Can you work these out from the model? Positions are in its coordinate system, mm. A direction names the side the tool comes from. Round coordinates to 2 decimals unless told otherwise and drop trailing zeros. Loops run counter-clockwise (first coordinate to the right, second up) from the corner with the lowest first, then second, coordinate; pieces in that order, holes last. Notation, with made-up numbers: (30.5, 20.25) -> (89.5, 20.25) arc R28 ccw to (89.5, 47.25) -> close; hole circle Ø6 at (-12.75, 51.25). An arc over 180 degrees is marked (long way). Use a Markdown table: item, result.
from build123d import *

# Parameters (mm, degrees)
PAD_DEPTH       = 86
SKETCH001_W     = 59.039818
SKETCH001_H     = 57
POCKET_DEPTH    = 56.001
SKETCH002_W     = 74.051056
SKETCH002_H     = 10
SKETCH002_W_2   = 70.317291
POCKET001_DEPTH = 51
SKETCH003_R     = 1.5
POCKET002_DEPTH = 5.001
SKETCH005_R     = 20
POCKET003_DEPTH = 30.001
SKETCH006_R     = 2.5
POCKET004_DEPTH = 30.001


with BuildPart() as part:
    # Sketch → Pad (new body)
    with BuildSketch(Plane.XZ):
        Polygon((0, 0), (30, 0), (30, 5), (5, 56), (0, 56), align=None)
    extrude(amount=PAD_DEPTH)

    # Sketch001 (on Face4 of Pad) → Pocket (cut, through all)
    with BuildSketch(Plane(origin=(0, 0, 56), x_dir=(-1, 0, 0), z_dir=(0, 0, 1))):
        with Locations((-34.519909, 43)):
            Rectangle(SKETCH001_W, SKETCH001_H)
    extrude(amount=-POCKET_DEPTH, mode=Mode.SUBTRACT)

    # Sketch002 (on Face11 of Pocket) → Pocket001 (cut)
    with BuildSketch(Plane(origin=(0, 0, 56), x_dir=(-1, 0, 0), z_dir=(0, 0, 1))):
        with Locations((-37.025528, 81)):
            Rectangle(SKETCH002_W, SKETCH002_H)
        with Locations((-35.158645, 5)):
            Rectangle(SKETCH002_W_2, SKETCH002_H)
    extrude(amount=-POCKET001_DEPTH, mode=Mode.SUBTRACT)

    # Sketch003 (on Face14 of Pocket001) → Pocket002 (cut, through all)
    with BuildSketch(Plane(origin=(0, 0, 5), x_dir=(-1, 0, 0), z_dir=(0, 0, 1))):
        with Locations((-20, 81)):
            Circle(SKETCH003_R)
        with Locations((-7.5, 81)):
            Circle(SKETCH003_R)
        with Locations((-20, 5)):
            Circle(SKETCH003_R)
        with Locations((-7.5, 5)):
            Circle(SKETCH003_R)
    extrude(amount=-POCKET002_DEPTH, mode=Mode.SUBTRACT)

    # Sketch005 (on Face3 of Pocket002) → Pocket003 (cut, through all)
    with BuildSketch(Plane(origin=(0, 0, 0), x_dir=(0, 0, -1), z_dir=(-1, 0, 0))):
        with Locations((-28, 43)):
            Circle(SKETCH005_R)
    extrude(amount=-POCKET003_DEPTH, mode=Mode.SUBTRACT)

    # Sketch006 (on Face3 of Pocket003) → Pocket004 (cut, through all)
    with BuildSketch(Plane(origin=(0, 0, 0), x_dir=(0, 0, -1), z_dir=(-1, 0, 0))):
        with Locations((-51.5, 66.5)):
            Circle(SKETCH006_R)
        with Locations((-4.5, 66.5)):
            Circle(SKETCH006_R)
        with Locations((-51.5, 19.5)):
            Circle(SKETCH006_R)
        with Locations((-4.5, 19.5)):
            Circle(SKETCH006_R)
    extrude(amount=-POCKET004_DEPTH, mode=Mode.SUBTRACT)


solid = part.part
1. Which directions (+Z, -Z, +X, -X, +Y, -Y) give clear straight access to the entire face, cutting with the end or side of a thin tool? Please do faces 5 (the flat face through (15, -14.5, 22)), 6 (the cylindrical face through (20.195, -82.487, 2.535)), 7 (the flat face through (9, -10, 25)).
Answer sheet:
| item | result |
|---|---|
| face 5 | +Z, -Z, +X |
| face 6 | +Z, -Z |
| face 7 | +Z, +X, -X, +Y |
2. I want a section at B-B (y = -43). Please give me the cut outline in (x, z), plus the area to 3 significant figures.
Answer sheet:
| item | result |
|---|---|
| outline | (0, 0) -> (5, 0) -> (5, 8) -> (0, 8) -> close; (0, 48) -> (5, 48) -> (5, 56) -> (0, 56) -> close |
| area | 80.0 mm² |
3. If we mould it in two halves opening along Z, with no side actions, what happens to faces 1 (the cylindrical face through (2.465, -49.007, 8.924)), 2 (the flat face through (17.675, -12.218, 30.143)), 3 (the flat face through (15, -71.5, 22)), 4 (the cylindrical face through (2.46, -65.54, 49.19))? For each: +Z half, -Z half, draft (parallel to the pull), parting line (faces both ways), or undercut.
Answer sheet:
| item | result |
|---|---|
| face 1 | undercut |
| face 2 | +Z half |
| face 3 | draft |
| face 4 | undercut |
4. I need wall thicknesses on line 1 (Y direction, x = 20, z = 2); line 2 (Y direction, x = 1.75, z = 51.5); line 3 (Y direction, x = 2.2, z = 4.5). Which ranges of each line are inside material? Lowest first, please.
Answer sheet:
| item | result |
|---|---|
| line 1 | y = -86 to -82.5, -79.5 to -71.5, -14.5 to -6.5, -3.5 to 0 |
| line 2 | y = -76 to -69, -64 to -22, -17 to -10 |
| line 3 | y = -86 to -69, -64 to -22, -17 to 0 |
5. I want a section at A-A (x = 15.5). Please give me the cut outline in (y, z).
Answer sheet:
| item | result |
|---|---|
| outline | (-86, 0) -> (-71.5, 0) -> (-71.5, 34.58) -> (-76, 34.58) -> (-76, 5) -> (-86, 5) -> close; (-14.5, 0) -> (0, 0) -> (0, 5) -> (-10, 5) -> (-10, 34.58) -> (-14.5, 34.58) -> close |
6. I want a section at C-C (y = -5). Please give me the cut outline in (x, z), plus the area to 3 significant figures.
Answer sheet:
| item | result |
|---|---|
| outline | (0, 0) -> (6, 0) -> (6, 5) -> (0, 5) -> close; (9, 0) -> (18.5, 0) -> (18.5, 5) -> (9, 5) -> close; (21.5, 0) -> (30, 0) -> (30, 5) -> (21.5, 5) -> close |
| area | 120 mm² |
7. I want a section at D-D (z = 6). Please give me the cut outline in (x, y).
Answer sheet:
| item | result |
|---|---|
| outline | (0, -76) -> (29.51, -76) -> (29.51, -71.5) -> (5, -71.5) -> (5, -68.5) -> (0, -68.5) -> close; (0, -64.5) -> (5, -64.5) -> (5, -21.5) -> (0, -21.5) -> close; (0, -17.5) -> (5, -17.5) -> (5, -14.5) -> (29.51, -14.5) -> (29.51, -10) -> (0, -10) -> close |
8. Will these pins go through, and if not, where does the flat tip stop? pin 1 Ø8 at (y, z) = (-19.5, 51.5) entering from +X; pin 2 Ø4 at (x, y) = (20, -81) entering from +Z; pin 3 Ø7.5 at (x, z) = (23.5, 22) entering from +Y.
Answer sheet:
| item | result |
|---|---|
| pin 1 | stops at x = 5 |
| pin 2 | stops at z = 5 |
| pin 3 | stops at y = -10 |
